Geometry: final body of the model. Coordinates: model frame, mm. Round coordinates to 2 decimals unless told otherwise and drop trailing zeros. Write each loop counter-clockwise with the first axis right and the second up, starting at its lowest first coordinate (ties: lowest second). Pieces come first, ordered by that corner, then holes. Notation, with made-up numbers: (12.25, 28.5) -> (46.25, 28.5) arc R22 ccw to (46.25, 67.5) -> close; hole circle Ø9 at (1.5, 42.25). An arc over 180 degrees is marked (long way). Use one line per item in the form item = value. Start each with the question number.
1. Cut plane A-A, the plane z = 7.5. Return the cut outline in (x, y), plus the area to 3 significant figures.
2. Cut plane D-D, the plane x = -18.5. State how many separate pieces and enclosed holes the cut face has, plus the area to 3 significant figures.
3. Line query: L1, parallel to X at y = 45, z = -6.5; L2, parallel to Y at x = 17.5, z = -9; L3, parallel to Y at x = -18, z = 4.75. Output: solid intervals per line, ascending.
4. Pin query (flat end, axial travel): pin 1 Ø8 at (y, z) = (146.5, 6.5) entering from +X; pin 2 Ø3 at (x, z) = (3.5, 6) entering from -Y; pin 3 Ø5.5 at (x, z) = (-91.5, -8.5) entering from -Y. Return the tip coordinate at first contact, or that it passes through.
5. Cut plane B-B, the plane x = 70.5. Return the cut outline in (y, z).
6. Cut plane C-C, the plane y = 50. Return the cut outline in (x, z).
Autodesk Inventor part; units mm, degrees
ref_plane "Work Plane1" through (0, 0, 0) normal (1, 0, 0) x (0, 1, 0)
ref_plane "Work Plane2" through (0, 107.5, 0) normal (0, 1, 0) x (-1, 0, 0)
ref_plane "Work Plane3" through (0, 0, 0) normal (0, 1, 0) x (-1, 0, 0)
sketch "Sketch1" plane through (0, 0, 0) normal (1, 0, 0) x (0, 1, 0)
  line L0 (215, 0) -> (0, 0)
  line L1 (0, 0) -> (0, -15)
  line L2 (0, -15) -> (215, -15)
  line L3 (215, -15) -> (215, 0)
  dimension "d0" = 15
  dimension "d1" = 215
extrude "Extrusion1" add sketch "Sketch1" along normal mid plane 170
sketch "Sketch2" plane through (85, 0, 0) normal (1, 0, 0) x (0, 0, -1)
  line L0 (15, 0) -> (15, 215)
  line L1 (15, 215) -> (0, 215)
  line L2 (15, 215) -> (10, 215)
  line L3 (10, 215) -> (10, 205)
  line L4 (10, 205) -> (15, 205)
  line L5 (15, 205) -> (15, 215)
  point P0 (0, 0)
  point P1 (12.5, 215)
  point P2 (12.5, 205)
  point P3 (15, 210)
  point P4 (10, 210)
  point P5 (15, 205)
  dimension "d4" = 10
  dimension "d5" = 5
sketch3d "3D Sketch1"
  line L0 (85, 215, -15) -> (-85, 215, -15)
  line L1 (-85, 215, -15) -> (-85, 0, -15)
  line L2 (-85, 0, -15) -> (85, 0, -15)
  line L3 (85, 0, -15) -> (85, 215, -15)
sweep "Sweep1" cut profiles "Sketch2" path "3D Sketch1"
ref_plane "Work Plane1" through (0, 0, 0) normal (1, 0, 0) x (0, 1, 0)
sketch "Sketch3" plane through (0, 0, 0) normal (1, 0, 0) x (0, 1, 0)
  line L0 (0, 0) -> (215, 0)
  line L1 (190, 0) -> (180, 0)
  line L2 (180, 0) -> (180, 10)
  line L3 (180, 10) -> (190, 0)
  point P0 (180, 5)
  dimension "d9" = 25
  dimension "d10" = 10
  dimension "d11" = 10
extrude "Extrusion2" add sketch "Sketch3" along normal mid plane 60
sketch "Sketch4" plane through (0, 0, 0) normal (1, 0, 0) x (0, 1, 0)
  line L0 (10, -15) -> (205, -15)
  line L1 (180, -15) -> (180, 5)
  line L2 (180, 5) -> (185, 0)
  line L3 (185, 0) -> (185, -15)
  line L4 (185, -15) -> (180, -15)
  line L5 (180, 10) -> (190, 0)
  point P0 (0, 0)
  dimension "d14" = 5
  dimension "d15" = 5
extrude "Extrusion3" cut sketch "Sketch4" along normal mid plane 50
pattern_linear "Rectangular Pattern1" count 5 spacing 10 along (0, -1, 0) of "Extrusion2", "Extrusion3"
sketch "Sketch5" plane through (85, 0, 0) normal (1, 0, 0) x (0, 0, -1)
  line L0 (10, 0) -> (10, 215)
  line L1 (10, 10) -> (10, 205)
  line L2 (10, 177.5) -> (5, 177.5)
  line L3 (5, 177.5) -> (5, 162.5)
  line L4 (5, 162.5) -> (10, 162.5)
  line L5 (10, 162.5) -> (10, 177.5)
  point P0 (0, 0)
  point P1 (7.5, 177.5)
  point P2 (10, 177.5)
  point P3 (7.5, 162.5)
  dimension "d22" = 5
  dimension "d23" = 15
  dimension "d39" = 52.5
extrude "Extrusion4" add sketch "Sketch5" along normal blind 15
sketch "Sketch6" plane through (85, 162.5, -5) normal (0, 0, 1) x (1, 0, 0)
  line L0 (0, 15) -> (15, 15)
  line L1 (15, 15) -> (15, 0)
  point P0 (-85, -162.5)
  point P1 (7.5, 7.5)
  point P2 (7.5, 15)
  point P3 (15, 7.5)
  dimension "d26" = 7.5
  dimension "d27" = 7.5
hole "Hole1" at (92.5, 170, -5) direction (0, 0, -1) diameter 4.134 depth 5
ref_plane "Work Plane2" through (0, 107.5, 0) normal (0, 1, 0) x (-1, 0, 0)
mirror "Mirror1" about plane through (0, 107.5, 0) normal (0, 1, 0) of "Extrusion4", "Hole1"
ref_plane "Work Plane3" through (0, 0, 0) normal (0, 1, 0) x (-1, 0, 0)
ref_plane "Work Plane5" through (0, 0, 0) normal (1, 0, 0) x (0, 1, 0)
mirror "Mirror2" about plane through (0, 0, 0) normal (1, 0, 0) of "Extrusion4", "Hole1", "Mirror1"
properties part number "caseDoor"
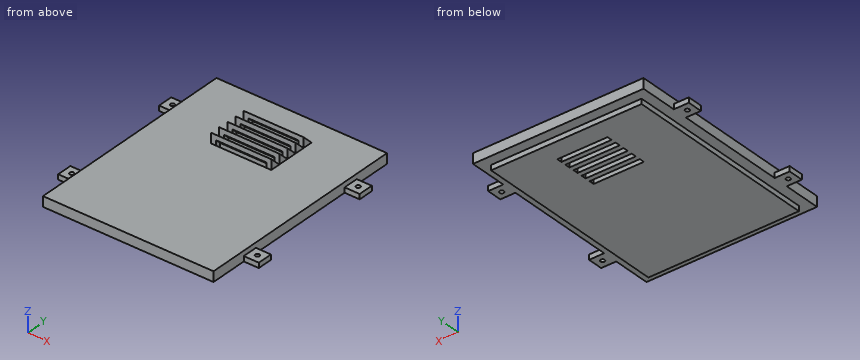
Outcome:
q1.outline = (-30, 140) -> (30, 140) -> (30, 142.5) -> (-30, 142.5) -> close; (-30, 150) -> (30, 150) -> (30, 152.5) -> (-30, 152.5) -> close; (-30, 160) -> (30, 160) -> (30, 162.5) -> (-30, 162.5) -> close; (-30, 170) -> (30, 170) -> (30, 172.5) -> (-30, 172.5) -> close; (-30, 180) -> (30, 180) -> (30, 182.5) -> (-30, 182.5) -> close
q1.area = 750 mm^2
q2.separate_pieces = 6
q2.enclosed_holes = 0
q2.area = 2,940 mm^2
q3.L1 = -100 to -94.57, -90.43 to 90.43, 94.57 to 100
q3.L2 = 0 to 140, 145 to 150, 155 to 160, 165 to 170, 175 to 180, 185 to 215
q3.L3 = 140.25 to 145.25, 150.25 to 155.25, 160.25 to 165.25, 170.25 to 175.25, 180.25 to 185.25
q4.pin_1 = 30
q4.pin_2 = 140
q4.pin_3 = 37.5
q5.outline = (0, -10) -> (10, -10) -> (10, -15) -> (205, -15) -> (205, -10) -> (215, -10) -> (215, 0) -> (0, 0) -> close
q6.outline = (-100, -10) -> (-75, -10) -> (-75, -15) -> (75, -15) -> (75, -10) -> (100, -10) -> (100, -5) -> (85, -5) -> (85, 0) -> (-85, 0) -> (-85, -5) -> (-100, -5) -> close
